Can you work these out from the model? Positions are in its coordinate system, mm. A direction names the side the tool comes from. Give positions to 0.01 mm unless a question says otherwise; leave off trailing zeros. Loops run counter-clockwise (first coordinate to the right, second up) from the corner with the lowest first, then second, coordinate; pieces in that order, holes last.
from build123d import *

# Parameters (mm, degrees)
SKETCH3_W           = 19.05
SKETCH3_H           = 19.05
SKETCH3_W_2         = 16.5608
SKETCH3_H_2         = 16.5608
BOSS_EXTRUDE1_DEPTH = 254.635
FILLET1_R           = 1.2446
SKETCH4_R           = 2.4892
CUT_EXTRUDE1_DEPTH  = 256.524189364
CUT_EXTRUDE3_START  = -19.05
CUT_EXTRUDE3_DEPTH  = 6.35
LPATTERN2_COUNT     = 8
LPATTERN2_PITCH     = 50.8


with BuildPart() as part:
    # Sketch3 → Boss-Extrude1 (new, symmetric)
    with BuildSketch(Plane.XY):
        Rectangle(SKETCH3_W, SKETCH3_H)
        Rectangle(SKETCH3_W_2, SKETCH3_H_2, mode=Mode.SUBTRACT)
    extrude(amount=BOSS_EXTRUDE1_DEPTH, both=True)

    # Fillet1
    fillet1_edges = [part.edges().sort_by_distance(p)[0] for p in [
        (-8.2804, -8.2804, 0),
        (8.2804, -8.2804, 0),
        (8.2804, 8.2804, 0),
        (-8.2804, 8.2804, 0),
        (9.525, -9.525, 0),
        (-9.525, -9.525, 0),
        (-9.525, 9.525, 0),
        (9.525, 9.525, 0),
    ]]
    fillet(fillet1_edges, radius=FILLET1_R)

    # Sketch4 → Cut-Extrude1 (cut, through all)
    with BuildSketch(Plane(origin=(0, 9.525, 0), x_dir=(1, 0, 0), z_dir=(0, 1, 0))):
        with Locations(Location((0, 159.385, 0), (0, 0, 270))):
            Circle(SKETCH4_R)
        with Locations(Location((0, 108.585, 0), (0, 0, 270))):
            Circle(SKETCH4_R)
        with Locations(Location((0, 57.785, 0), (0, 0, 270))):
            Circle(SKETCH4_R)
        with Locations(Location((0, 6.985, 0), (0, 0, 270))):
            Circle(SKETCH4_R)
        with Locations(Location((0, -43.815, 0), (0, 0, 270))):
            Circle(SKETCH4_R)
        with Locations(Location((0, -94.615, 0), (0, 0, 270))):
            Circle(SKETCH4_R)
        with Locations(Location((0, -145.415, 0), (0, 0, 270))):
            Circle(SKETCH4_R)
        with Locations(Location((0, -196.215, 0), (0, 0, 270))):
            Circle(SKETCH4_R)
    extrude(amount=-CUT_EXTRUDE1_DEPTH, mode=Mode.SUBTRACT)

    # Sketch6 → Cut-Extrude3 (cut)
    with BuildSketch(Plane.ZY.offset(9.525).offset(CUT_EXTRUDE3_START)):
        Polygon((-182.118, -1.651), (-187.198, -1.651), (-187.198, 9.525), (-192.278, 9.525), (-192.278, -6.477), (-182.118, -6.477), (-177.292, -6.477), (-177.292, -1.651), align=None)
    cut_extrude3 = extrude(amount=CUT_EXTRUDE3_DEPTH, mode=Mode.SUBTRACT)

    # LPattern2: Cut-Extrude3 ×8
    with Locations(*[(0, 0, i * LPATTERN2_PITCH) for i in range(1, LPATTERN2_COUNT)]):
        add(cut_extrude3, mode=Mode.SUBTRACT)


solid = part.part
(1) Which directions (+Z, -Z, +X, -X, +Y, -Y) give clear straight access to the entire face, cutting with the end or side of a thin tool? Please do faces 1 (the flat face through (-9, 0, 254.635)), 2 (the flat face through (0, -8.28, 4)).
Returned:
face 1: +Z, +X, -X, +Y, -Y
face 2: +Z, -Z
(2) Suppose I cut it at A-A on z = -97. List the corners of the cut face in (x, y) for me (3 decimals), plus the area to 3 significant figures.
Returned:
outline: (-9.525, -8.28) arc R1.245 ccw to (-8.28, -9.525) - (8.28, -9.525) arc R1.245 ccw to (9.525, -8.28) - (9.525, 8.28) arc R1.245 ccw to (8.28, 9.525) - (-8.28, 9.525) arc R1.245 ccw to (-9.525, 8.28) - close; hole (-8.28, -7.036) arc R1.245 ccw to (-7.036, -8.28) - (7.036, -8.28) arc R1.245 ccw to (8.28, -7.036) - (8.28, 7.036) arc R1.245 ccw to (7.036, 8.28) - (-7.036, 8.28) arc R1.245 ccw to (-8.28, 7.036) - close
area: 88.6 mm2
(3) Will these pins go through, and if not, where does the flat tip stop? P1, Ø0.6, axis at y = 9, z = 164.5, coming from the +X side (3 decimals); P2, Ø2, axis at x = 6, y = 3.5, coming from the +Z side; P3, Ø0.6, axis at x = 9, z = 14.5, coming from the +Y side; P4, Ø1, axis at x = 9, z = -33, coming from the +Y side.
Returned:
P1: stops at x = 3.175
P2: passes through
P3: stops at y = -6.48
P4: stops at y = 9.51
(4) Thinking about a two-plate mould opening in Y: for faces 3 (the flat face through (-9, 0, -254.635)), 4 (the flat face through (-8.28, 0, 4)), 5 (the flat face through (0, -9.525, 4)), 6 (the flat face through (0, 9.525, 4)), which applies, pulls with the +Y half, pulls with the -Y half, needs draft (parallel to the pull), parting line crosses it, or undercut?
Returned:
face 3: needs draft
face 4: undercut
face 5: pulls with the -Y half
face 6: pulls with the +Y half
(5) Please list where these lines run through material, in increasing order: probe 1 along X at (y, z) = (-2.5, 143) (3 decimals); probe 2 along Y at (x, z) = (8.75, 76).
Returned:
probe 1: x = -9.525 to -8.28, 8.28 to 9.525
probe 2: y = -9.43 to -6.48, -1.65 to 9.43
